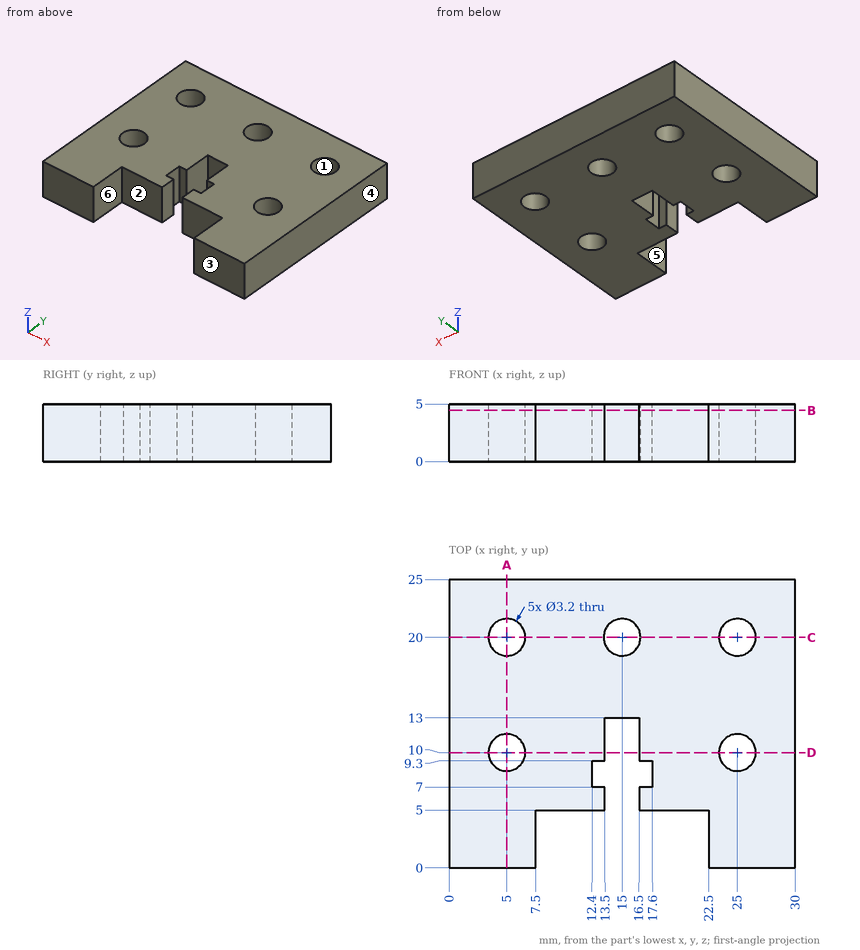
The figure shows three views and two pictorial views of one solid part (mm, origin at its lowest corner). Answer the questions. A direction names the side the tool comes from. Coordinates: 2 decimals unless noted, no trailing zeros. Order: outer loops, then holes, each group sorted by start corner. A loop starts at its lowest first (then second) coordinate and runs counter-clockwise, first axis right, second up. Notation, with made-up numbers: M 47,85.25 L 75,85.25 A26 ccw 75,106.25 Z; hole C -15.5,0.25 d1. An arc over 180 degrees is marked long. Use CSV: the item, a comma, the result in double quotes.
1) Section A-A on x = 5 is taken. Write down the section's boundary in (y, z).
Worked out:
outline,"M 0,0 L 8.4,0 L 8.4,5 L 0,5 Z; M 11.6,0 L 18.4,0 L 18.4,5 L 11.6,5 Z; M 21.6,0 L 25,0 L 25,5 L 21.6,5 Z"
2) Determine the mould class of the marked faces 3, 4, 5 and 6 for opening direction X: released by +X, released by -X, zero draft, split by the parting line, or undercut.
Worked out:
face 3,"zero draft"
face 4,"released by +X"
face 5,"undercut"
face 6,"undercut"
3) For the marked faces 1 and 2, determine the directions among +Z, -Z, +X, -X, +Y, -Y from which every point of the face is accessible in a straight line to the end or side of a thin tool.
Worked out:
face 1,"+Z, -Z"
face 2,"+Z, -Z, -Y"
4) Section C-C on y = 20 is taken. Write down the section's boundary in (x, z).
Worked out:
outline,"M 0,0 L 3.4,0 L 3.4,5 L 0,5 Z; M 6.6,0 L 13.4,0 L 13.4,5 L 6.6,5 Z; M 16.6,0 L 23.4,0 L 23.4,5 L 16.6,5 Z; M 26.6,0 L 30,0 L 30,5 L 26.6,5 Z"
5) Section D-D on y = 10 is taken. Write down the section's boundary in (x, z).
Worked out:
outline,"M 0,0 L 3.4,0 L 3.4,5 L 0,5 Z; M 6.6,0 L 13.5,0 L 13.5,5 L 6.6,5 Z; M 16.5,0 L 23.4,0 L 23.4,5 L 16.5,5 Z; M 26.6,0 L 30,0 L 30,5 L 26.6,5 Z"
6) Flat-ended cylindrical pins translate along their axes: pin 1 Ø5 at (x, y) = (25, 10) entering from +Z; pin 2 Ø0.9 at (x, z) = (15.5, 2) entering from -Y; pin 3 Ø0.6 at (x, z) = (17.5, 3.5) entering from -Y. Find the tip coordinate at first contact, or state that the pin passes through.
Worked out:
pin 1,"stops at z = 5"
pin 2,"stops at y = 13"
pin 3,"stops at y = 5"
7) Consider line 1 (Y direction, x = 25, z = 2.8); line 2 (X direction, y = 10.75, z = 3.05); line 3 (Y direction, x = 19.5, z = 0.35). Determine where each line is inside the solid, lowest interval first. Write a range as [from, to].
Worked out:
line 1,"y = [0, 8.4], [11.6, 18.4], [21.6, 25]"
line 2,"x = [0, 3.59], [6.41, 13.5], [16.5, 23.59], [26.41, 30]"
line 3,"y = [5, 25]"
8) Section B-B on z = 4.45 is taken. Write down the section's boundary in (x, y).
Worked out:
outline,"M 0,0 L 7.5,0 L 7.5,5 L 13.5,5 L 13.5,7 L 12.4,7 L 12.4,9.3 L 13.5,9.3 L 13.5,13 L 16.5,13 L 16.5,9.3 L 17.6,9.3 L 17.6,7 L 16.5,7 L 16.5,5 L 22.5,5 L 22.5,0 L 30,0 L 30,25 L 0,25 Z; hole C 5,10 d3.2; hole C 5,20 d3.2; hole C 15,20 d3.2; hole C 25,10 d3.2; hole C 25,20 d3.2"
